Geometry check sheet. Reference: the model listing, model coordinates, mm. A direction names the side the tool comes from. Give positions to 0.01 mm unless a question says otherwise; leave off trailing zeros. Loops run counter-clockwise (first coordinate to the right, second up) from the corner with the lowest first, then second, coordinate; pieces in that order, holes last. Notation, with made-up numbers: (31.25, 86.25) -> (82.25, 86.25) arc R28 cw to (82.25, 117.25) -> close; hole circle Ø10 at (-13.5, 34). An arc over 180 degrees is marked (long way). Write each question's results on one line, items separated by ' | '. Start each with the question number.
1) Scan lines: line 1 (Z direction, x = 23.5, y = 46.5); line 2 (Y direction, x = 25, z = 47); line 3 (Y direction, x = 7, z = -26.5). Record each from-to range of solid material in increasing order. Write a range as from..to.
2) Depth check by flat-ended pin: pin 1 (8 mm diameter, centred on x = 51, z = 30.5, fed in from -Y); pin 2 (24 mm diameter, centred on x = 25.5, y = 70, fed in from +Z). Enter the tip coordinate at first touch or a pass-through.
3) Sectioned sample at D-D on y = 36. Record the cut outline in (x, z), then the cut area to 3 significant figures.
4) Sectioned sample at B-B on z = 37.5. Record the cut outline in (x, y), then the cut area to 3 significant figures.
5) Sectioned sample at C-C on x = 82.5. Record the cut outline in (y, z), then the cut area to 3 significant figures.
6) Sectioned sample at A-A on x = 25.5. Record the cut outline in (y, z).
7) Draft check along X on faces 4 (the face through (19.95, 94.89, 42.6)), 5 (the face through (50, 38, 50)), 6 (the face through (28.752, 55.357, -42.605)). Enter one of: pulls with the +X half, pulls with the -X half, needs draft (parallel to the pull), parting line crosses it, or undercut.
8) Set-up check for faces 1 (the face through (28.752, 55.357, 42.395)), 2 (the face through (31, 49, 35)), 3 (the face through (99, 10, -20)): record each of +Z, -Z, +X, -X, +Y, -Y from which the full face is reachable in a straight line by a thin tool's end or side.
```python
from build123d import *

# Parameters (mm, degrees)
BOSS_EXTRUDE1_DEPTH    = 50
SKETCH2_W              = 171.937170065
SKETCH2_H              = 70
CUT_EXTRUDE1_DEPTH     = 159.430584169
CUT_EXTRUDE2_DEPTH     = 159.430584169
F_20_0MM_DOWEL_HOLE1_D = 30


with BuildPart() as part:
    # Sketch1 → Boss-Extrude1 (new, symmetric)
    with BuildSketch(Plane.XY):
        with BuildLine():
            Line((0, 0), (130, 0))
            Line((130, 0), (110, 20))
            Line((110, 20), (80, 20))
            Line((80, 20), (48.160217592, 81.694637176))
            ThreePointArc((48.160217592, 81.694637176), (19.482755972, 94.779886487), (0, 70))
            Line((0, 70), (0, 0))
        make_face()
    extrude(amount=BOSS_EXTRUDE1_DEPTH, both=True)

    # Sketch2 → Cut-Extrude1 (cut, through all)
    with BuildSketch(Plane(origin=(0, 20, 0), x_dir=(1, 0, 0), z_dir=(0, 1, 0))):
        with Locations((69.738425947, 0)):
            Rectangle(SKETCH2_W, SKETCH2_H)
    extrude(amount=CUT_EXTRUDE1_DEPTH, mode=Mode.SUBTRACT)

    # Sketch3 → Cut-Extrude2 (cut, through all)
    with BuildSketch(Plane(origin=(0, 20, 0), x_dir=(1, 0, 0), z_dir=(0, 1, 0))):
        with BuildLine():
            Line((80, 20), (153.648677571, 20))
            Line((153.648677571, 20), (153.648677571, -20))
            Line((153.648677571, -20), (80, -20))
            ThreePointArc((80, -20), (60, 0), (80, 20))
        make_face()
    extrude(amount=-CUT_EXTRUDE2_DEPTH, mode=Mode.SUBTRACT)

    # Ø20.0mm Dowel Hole1 (through all)
    with Locations(Plane.XY.offset(50)):
        with Locations((25.5, 70)):
            Hole(F_20_0MM_DOWEL_HOLE1_D / 2)


solid = part.part
```
Result:
1) line 1: -50..-35, 35..50 | line 2: 0..55.01, 84.99..95.5 | line 3: 0..20
2) pin 1: y = 0 | pin 2: through
3) outline: (0, -50) -> (71.74, -50) -> (71.74, -35) -> (0, -35) -> close; (0, 35) -> (71.74, 35) -> (71.74, 50) -> (0, 50) -> close | area: 2,150 mm^2
4) outline: (0, 0) -> (130, 0) -> (110, 20) -> (80, 20) -> (48.16, 81.69) arc R25.5 ccw to (0, 70) -> close; hole circle Ø30 at (25.5, 70) | area: 6,080 mm^2
5) outline: (0, -50) -> (20, -50) -> (20, -20) -> (0, -20) -> close; (0, 20) -> (20, 20) -> (20, 50) -> (0, 50) -> close | area: 1,200 mm^2
6) outline: (0, -50) -> (55, -50) -> (55, -35) -> (20, -35) -> (20, 35) -> (55, 35) -> (55, 50) -> (0, 50) -> close; (85, -50) -> (95.5, -50) -> (95.5, -35) -> (85, -35) -> close; (85, 35) -> (95.5, 35) -> (95.5, 50) -> (85, 50) -> close
7) face 4: parting line crosses it | face 5: needs draft | face 6: undercut
8) face 1: +Z, -Z | face 2: +X, -X, +Y | face 3: +X, +Y, -Y
